from build123d import *
from build123d.topology import SkipClean

# Parameters (mm, degrees)
BOSS_EXTRUDE1_DEPTH      = 0.5
BOSS_EXTRUDE1_DEPTH_BACK = 0.5
SKETCH1_R                = 3.5
CUT_EXTRUDE1_DEPTH       = 14.5


with BuildPart() as part:
    # Sketch1 → Boss-Extrude1 (new, two sides: drawn at the far end of the back side and taken through both)
    with BuildSketch(Plane(origin=(0, 0, 0), x_dir=(1, 0, 0), z_dir=(0, 1, 0)).offset(-BOSS_EXTRUDE1_DEPTH_BACK)):
        with BuildLine():
            Line((-24, 25), (24, 25))
            ThreePointArc((24, 25), (24.707106781, 24.707106781), (25, 24))
            Line((25, 24), (25, -24))
            ThreePointArc((25, -24), (24.707106781, -24.707106781), (24, -25))
            Line((24, -25), (-24, -25))
            ThreePointArc((-24, -25), (-24.707106781, -24.707106781), (-25, -24))
            Line((-25, -24), (-25, 24))
            ThreePointArc((-25, 24), (-24.707106781, 24.707106781), (-24, 25))
        make_face()
        with Locations(Location((0, 0, 0), (0, 0, 270))):
            Circle(SKETCH1_R, mode=Mode.SUBTRACT)
    extrude(amount=BOSS_EXTRUDE1_DEPTH + BOSS_EXTRUDE1_DEPTH_BACK)

    # Sketch2 → Revolve1 (revolve)
    with SkipClean():  # the faces are left unmerged after this step: merging them gives an invalid solid
        with BuildSketch(Plane.XY, mode=Mode.PRIVATE) as revolve1_sk:
            Polygon((-8, 15), (-10, 15), (-17.5, 0.5), (-3.5, 0.5), (-3.5, 10), (-8, 10), align=None)
        revolve(revolve1_sk.sketch.rotate(Axis((0, 0.5, 0), (0, 1, 0)), 180), axis=Axis((0, 0.5, 0), (0, 1, 0)))
    add(part.part.scale(1), mode=Mode.REPLACE)  # the faces are merged on a copy

    # Sketch4 → Cut-Extrude1 (cut)
    with BuildSketch(Plane(origin=(0, 15, 0), x_dir=(1, 0, 0), z_dir=(0, 1, 0))):
        with BuildLine():
            Line((25, -0.324292046), (-1.009690159, -4.582097133))
            ThreePointArc((-1.009690159, -4.582097133), (-6.229441906, -11.256511144), (0, -17))
            Line((0, -17), (25, -17))
            Line((25, -17), (25, -7.125))
            Line((25, -7.125), (25, -0.324292046))
        make_face()
    extrude(amount=-CUT_EXTRUDE1_DEPTH, mode=Mode.SUBTRACT)


solid = part.part
Can you work these out from the model? Positions are in its coordinate system, mm. A direction names the side the tool comes from. Give positions to 0.01 mm unless a question says otherwise; leave off trailing zeros. Loops run counter-clockwise (first coordinate to the right, second up) from the corner with the lowest first, then second, coordinate; pieces in that order, holes last. Notation, with made-up numbers: (74, -35.5) -> (103, -35.5) arc R9 cw to (103, -21.5) -> close; hole circle Ø4 at (-16, 42). An arc over 180 degrees is marked (long way). Use one line per item in the form item = value.
1) Will these pins go through, and if not, where does the flat tip stop? pin 1 (0.5 mm diameter, centred on x = 2, y = 1, fed in from -Z); pin 2 (6 mm diameter, centred on x = 13, y = 8.5, fed in from -Z); pin 3 (5 mm diameter, centred on x = 12.5, y = 7, fed in from -Z); pin 4 (6.5 mm diameter, centred on x = 0, z = 0, fed in from -Y).
Answers:
pin_1 = -17.26
pin_2 = -9.59
pin_3 = -10.59
pin_4 = through
2) If we section it at D-D (y = 11.75): Please give me the cut outline in (x, z).
Answers:
outline = (-6.19, 9.9) arc R11.68 ccw (long way) to (11.4, 2.55) -> (7.32, 3.22) arc R8 cw (long way) to (-4.61, 6.53) arc R6.25 cw to start
3) If we section it at B-B (y = 2.5): Please give me the cut outline in (x, z), plus the area to 3 significant figures.
Answers:
outline = (-3.12, 16.17) arc R16.47 ccw (long way) to (16.37, 1.74) -> (-1.01, 4.58) arc R6.25 cw to start; hole circle Ø7 at (0, 0)
area = 591 mm²
4) I need wall thicknesses on line 1 along X through (y, z) = (12.4, 0); line 2 along Y through (x, z) = (7.5, 0.5); line 3 along Z through (x, y) = (0, 7). Which ranges of each line are inside material? Lowest first, please.
Answers:
line_1 = -11.34 to -8, 8 to 11.34
line_2 = -0.5 to 10
line_3 = -14.14 to -3.5, 3.5 to 4.42
5) For faces 1 (the face through (-6, 6, 9)), 2 (the face through (-1.4, 15, -8.4)), 3 (the face through (0, 10, -4)), which set-ups out of +Z, -Z, +X, -X, +Y, -Y let a thin tool reach every point of the face, with its end or its side?
Answers:
face_1 = +X, +Y
face_2 = +Z, -Z, +X, -X, +Y
face_3 = +Y
6) If we section it at A-A (z = 0): Please give me the cut outline in (x, y), plus the area to 3 significant figures.
Answers:
outline = (-25, -0.5) -> (-3.5, -0.5) -> (-3.5, 10) -> (-8, 10) -> (-8, 15) -> (-10, 15) -> (-17.5, 0.5) -> (-25, 0.5) -> close; (3.5, -0.5) -> (25, -0.5) -> (25, 0.5) -> (17.5, 0.5) -> (10, 15) -> (8, 15) -> (8, 10) -> (3.5, 10) -> close
area = 295 mm²
7) If we section it at C-C (x = 19.5): Please give me the cut outline in (y, z).
Answers:
outline = (-0.5, -25) -> (0.5, -25) -> (0.5, 25) -> (-0.5, 25) -> close
